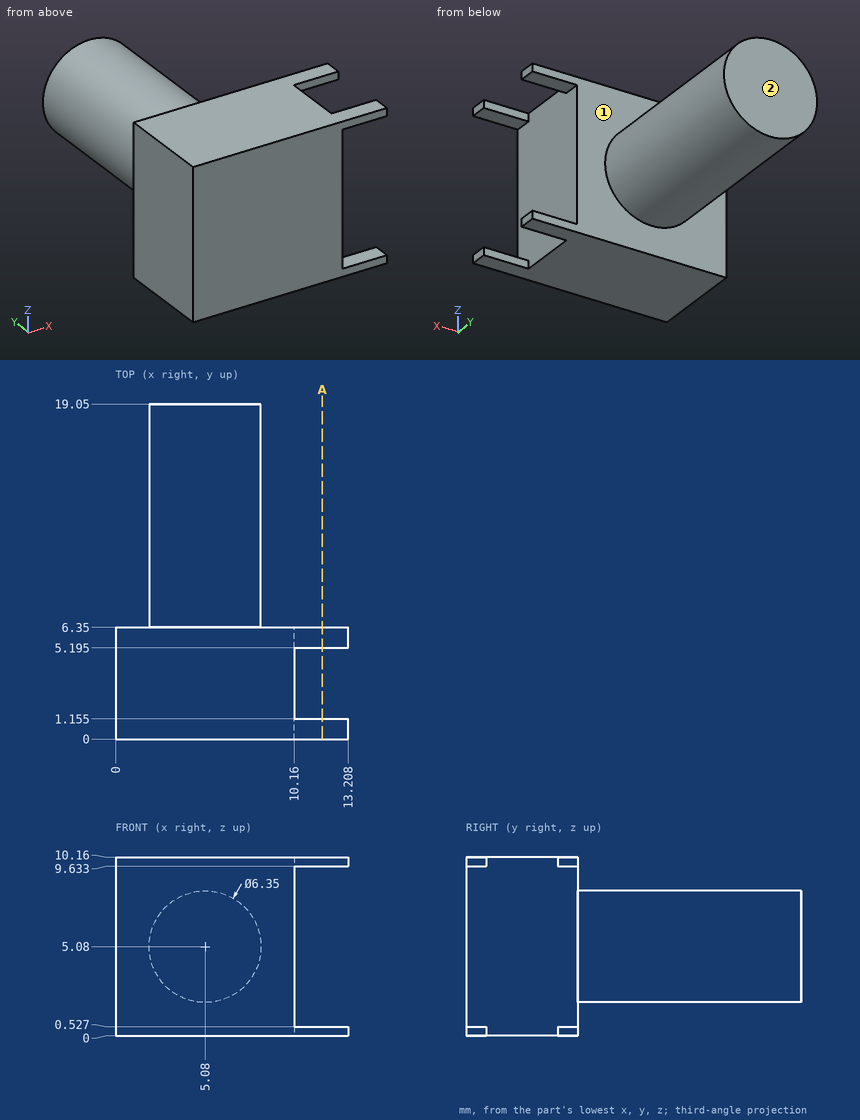
Print and shaded views of the part. All mm, measured from the part's lowest x, y and z. A direction names the side the tool comes from. Round coordinates to 2 decimals unless told otherwise and drop trailing zeros. Use a Markdown table: item, result. Add a question column.
1. 3-axis set-ups, long thin cutter, end or side, ignore diameter. For the marked faces 1 and 2: which of +Z, -Z, +X, -X, +Y, -Y reach the whole face in a straight line?
2. Drill centre lines: probe 1 along Z at (x, y) = (12, 5.5); probe 2 along Y at (x, z) = (1, 9); probe 3 along X at (y, z) = (4.25, 4.5). Where is each one in solid material? Low to high.
3. Flat gauge pins, fed straight in: P1, Ø4, axis at y = 6.5, z = 3, coming from the +X side; P2, Ø4, axis at x = 1.5, y = 12.5, coming from the +Z side (1 decimal); P3, Ø3, axis at x = 2.5, y = 15, coming from the +Z side (1 decimal); P4, Ø3, axis at x = 8.5, z = 4.5, coming from the +Y side. Where does each tip first touch, or does it go through?
4. Slice it at A-A on x = 11.75. Give the number of separate pieces and of enclosed holes in the cut face.
Reply:
| question | item | result |
|---|---|---|
| 1 | face 1 | +Y |
| 1 | face 2 | +Z, -Z, +X, -X, +Y |
| 2 | probe 1 | z = 0 to 0.53, 9.63 to 10.16 |
| 2 | probe 2 | y = 0 to 6.35 |
| 2 | probe 3 | x = 0 to 10.16 |
| 3 | P1 | stops at x = 10.16 |
| 3 | P2 | stops at z = 7.8 |
| 3 | P3 | stops at z = 8.1 |
| 3 | P4 | stops at y = 19.05 |
| 4 | separate pieces | 4 |
| 4 | enclosed holes | 0 |
